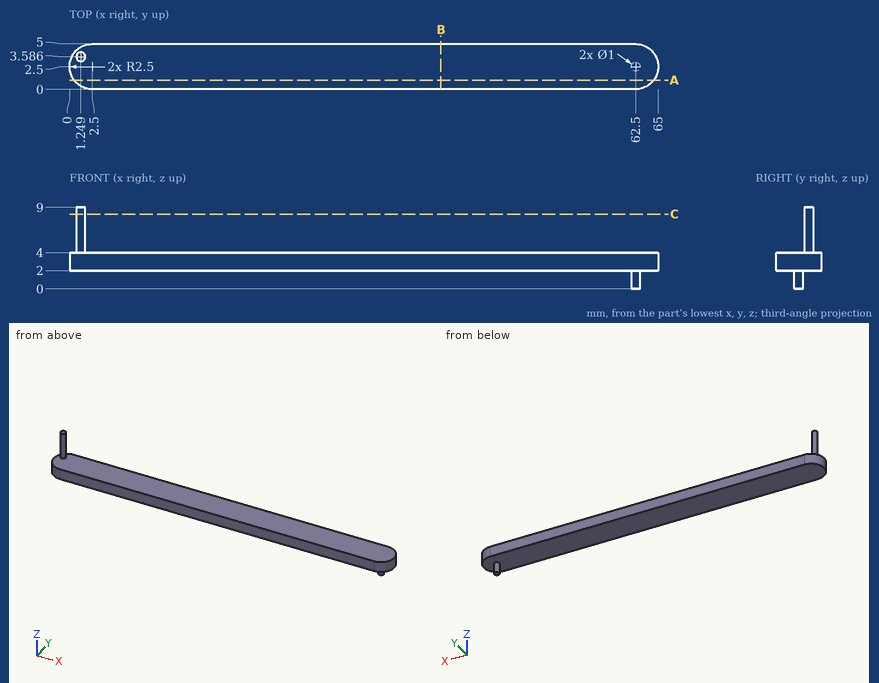
Print and shaded views of the part. All mm, measured from the part's lowest x, y and z. Give positions to 0.01 mm unless a question says otherwise; leave off trailing zeros. Loops run counter-clockwise (first coordinate to the right, second up) from the corner with the lowest first, then second, coordinate; pieces in that order, holes last.
1) Wall check: line 1 (Z direction, x = 56, y = 0.4); line 2 (X direction, y = 3.95, z = 7.5) (1 decimal); line 3 (X direction, y = 4, z = 8.25) (1 decimal). Give the ranges that are in metal, low to high.
2) Saw through at A-A (y = 1). Write the cut outline in (x, z), plus the area to 3 significant figures.
3) Saw through at B-B (x = 41). Write the cut outline in (y, z).
4) Flat gauge pins, fed straight in: pin 1 Ø1.5 at (x, y) = (23, 2) entering from -Z; pin 2 Ø1 at (x, y) = (13, 1.5) entering from +Z; pin 3 Ø1.5 at (x, z) = (48.5, 6.5) entering from -Y. Where does each tip first touch, or does it go through?
5) Saw through at C-C (z = 8.25). Write the cut outline in (x, y).
Answer block:
1. line 1: z = 2 to 4
1. line 2: x = 0.9 to 1.6
1. line 3: x = 1 to 1.5
2. outline: (0.5, 2) - (64.5, 2) - (64.5, 4) - (0.5, 4) - close
2. area: 128 mm2
3. outline: (0, 2) - (5, 2) - (5, 4) - (0, 4) - close
4. pin 1: stops at z = 2
4. pin 2: stops at z = 4
4. pin 3: passes through
5. outline: circle Ø1 at (1.25, 3.59)
